Design review of the part shown in the three views and the two pictorial views. Dimensions are in mm from the part's minimum x, y and z. Coordinates: 2 decimals unless noted, no trailing zeros. Loops run counter-clockwise (first coordinate to the right, second up) from the corner with the lowest first, then second, coordinate; pieces in that order, holes last. Notation, with made-up numbers: (42, -39) -> (89, -39) arc R21 ccw to (89, -35) -> close; hole circle Ø1 at (17.25, 15.25). An arc over 180 degrees is marked (long way). Use a Markdown table: item, result. Add a question column.
Q1. Draft analysis for pull direction X (two halves, no side actions). For the marked faces 1 and 2, state which applies: pulls with the +X half, pulls with the -X half, needs draft (parallel to the pull), parting line crosses it, or undercut.
Q2. Take a section at B-B on x = 86. Write out the cut boundary in (y, z).
Q3. Take a section at A-A on z = 3.3. Write out the cut boundary in (x, y).
Q4. For probe 1 along Y at (x, z) = (78, 2.65); probe 2 along X at (y, z) = (7, 2.4); probe 3 along Z at (x, y) = (20, 47), list the stretches that pass through material, from the lowest coordinate up.
Q5. Take a section at C-C on y = 44. Write out the cut boundary in (x, z).
Q6. Clearance check with flat-ended pins moving along their axes: pin 1 Ø1.6 at (y, z) = (47.5, 3.5) entering from -X; pin 2 Ø0.6 at (x, z) = (75, 3) entering from -Y; pin 3 Ø1.6 at (x, z) = (35, 3) entering from +Y. State where each tip first meets the part, or that it passes through.
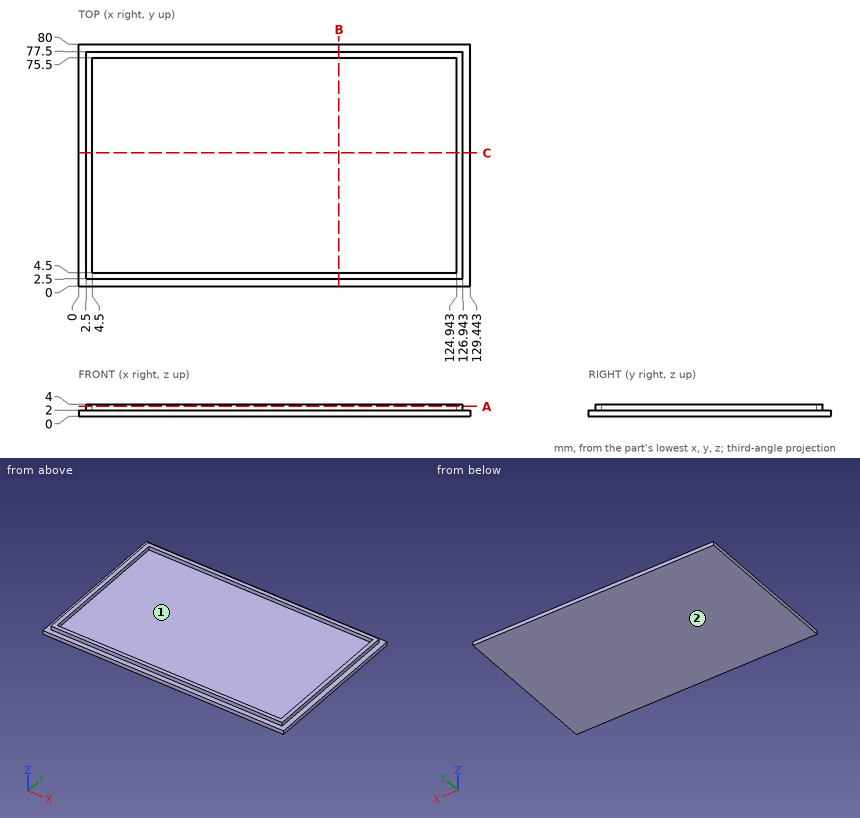
Answer list:
| question | item | result |
|---|---|---|
| 1 | face 1 | undercut |
| 1 | face 2 | needs draft |
| 2 | outline | (0, 0) -> (80, 0) -> (80, 2) -> (77.5, 2) -> (77.5, 4) -> (75.5, 4) -> (75.5, 2) -> (4.5, 2) -> (4.5, 4) -> (2.5, 4) -> (2.5, 2) -> (0, 2) -> close |
| 3 | outline | (2.5, 2.5) -> (126.94, 2.5) -> (126.94, 77.5) -> (2.5, 77.5) -> close; hole (4.5, 4.5) -> (124.94, 4.5) -> (124.94, 75.5) -> (4.5, 75.5) -> close |
| 4 | probe 1 | 2.5 to 4.5, 75.5 to 77.5 |
| 4 | probe 2 | 2.5 to 4.5, 124.94 to 126.94 |
| 4 | probe 3 | 0 to 2 |
| 5 | outline | (0, 0) -> (129.44, 0) -> (129.44, 2) -> (126.94, 2) -> (126.94, 4) -> (124.94, 4) -> (124.94, 2) -> (4.5, 2) -> (4.5, 4) -> (2.5, 4) -> (2.5, 2) -> (0, 2) -> close |
| 6 | pin 1 | x = 2.5 |
| 6 | pin 2 | y = 2.5 |
| 6 | pin 3 | y = 77.5 |
